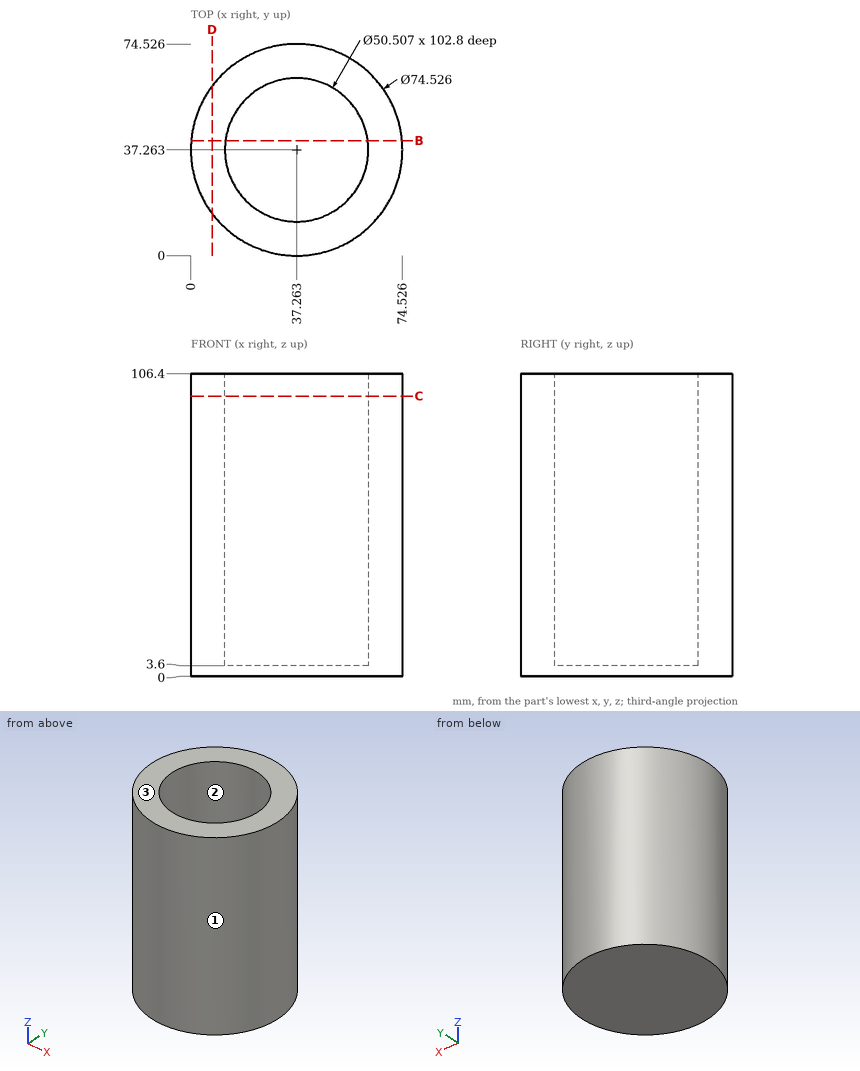
For this review, use the dimensioned drawing (mm, ordinates from the lowest corner) and the shaded views. Give positions to 0.01 mm unless a question says otherwise; leave off trailing zeros. Order: outer loops, then holes, each group sorted by start corner. A loop starts at its lowest first (then second) coordinate and runs counter-clockwise, first axis right, second up. Notation, with made-up numbers: (-20.75, -26) - (7.25, -26) arc R11 ccw to (7.25, -16) - close; hole circle Ø10 at (25, 53). An arc over 180 degrees is marked (long way). Use CSV: the item, a comma, the result in double quotes. Start each with the question number.
Q1. Take a section at C-C (z = 98.5). State the section outline as (x, y) points.
Q2. Draft analysis for pull direction X (two halves, no side actions). For the marked faces 1, 2 and 3, state which applies: pulls with the +X half, pulls with the -X half, needs draft (parallel to the pull), parting line crosses it, or undercut.
Q3. For P1, Ø5, axis at y = 64, z = 61.5, coming from the +X side; P2, Ø10, axis at x = 12.5, y = 10, coming from the -Z side; P3, Ø3, axis at y = 52, z = 47, coming from the +X side (1 decimal); P4, Ø2, axis at y = 12.5, z = 76, coming from the -X side, all flat-tipped, find the tip position at first contact; note any pin that passes through.
Q4. Take a section at D-D (x = 7.5). State the section outline as (y, z) points, and give its area (3 significant figures).
Q5. Take a section at B-B (y = 40.5). State the section outline as (x, z) points (1 decimal).
Q6. For line 1 (Z direction, x = 37.5, y = 51.5); line 2 (Y direction, x = 41, z = 71); line 3 (Y direction, x = 39, z = 30) (1 decimal), list the stretches that pass through material, from the lowest coordinate up.
Calculated:
1,outline,"circle Ø74.53 at (37.26, 37.26); hole circle Ø50.51 at (37.26, 37.26)"
2,face 1,"parting line crosses it"
2,face 2,"undercut"
2,face 3,"needs draft"
3,P1,"stops at x = 65.57"
3,P2,"stops at z = 0"
3,P3,"stops at x = 72.1"
3,P4,"stops at x = 8.56"
4,outline,"(14.84, 0) - (59.68, 0) - (59.68, 106.4) - (14.84, 106.4) - close"
4,area,"4,770 mm²"
5,outline,"(0.1, 0) - (74.4, 0) - (74.4, 106.4) - (62.3, 106.4) - (62.3, 3.6) - (12.2, 3.6) - (12.2, 106.4) - (0.1, 106.4) - close"
6,line 1,"z = 0 to 3.6"
6,line 2,"y = 0.19 to 12.29, 62.24 to 74.34"
6,line 3,"y = 0 to 12.1, 62.5 to 74.5"
